from build123d import *

# Parameters (mm, degrees)
SKETCH1_W               = 83.0326
SKETCH1_H               = 17.653
BOSS_EXTRUDE1_DEPTH     = 6.3119
SKETCH5_W               = 2.286
SKETCH5_H               = 21.717
BOSS_EXTRUDE5_DEPTH     = 10.8712
LPATTERN2_COUNT         = 8
LPATTERN2_PITCH         = 9.445171429
SKETCH9_R               = 2.032
CUT_EXTRUDE1_DEPTH      = 86.567236542
MIRROR2_COPY_1_SKETCH_R = 2.032
MIRROR2_COPY_1_DEPTH    = 86.567236542


with BuildPart() as part:
    # Sketch1 → Boss-Extrude1 (new body)
    with BuildSketch(Plane(origin=(0, 0, 0), x_dir=(1, 0, 0), z_dir=(0, 1, 0))):
        with Locations((41.5163, 8.8265)):
            Rectangle(SKETCH1_W, SKETCH1_H)
    extrude(amount=BOSS_EXTRUDE1_DEPTH)

    # Sketch5 → Boss-Extrude5 (add)
    with BuildSketch(Plane.XZ):
        with Locations((8.4582, -8.8265)):
            Rectangle(SKETCH5_W, SKETCH5_H)
    boss_extrude5 = extrude(amount=-BOSS_EXTRUDE5_DEPTH)

    # LPattern2: Boss-Extrude5 ×8
    with Locations(*[(i * LPATTERN2_PITCH, 0, 0) for i in range(1, LPATTERN2_COUNT)]):
        add(boss_extrude5)

    # Sketch9 → Cut-Extrude1 (cut, through all)
    with BuildSketch(Plane(origin=(0, 6.3119, 0), x_dir=(1, 0, 0), z_dir=(0, 1, 0))):
        with Locations(Location((3.3401, 5.08, 0), (0, 0, 270))):
            Circle(SKETCH9_R)
    cut_extrude1 = extrude(amount=-CUT_EXTRUDE1_DEPTH, mode=Mode.SUBTRACT)

    # Mirror1: Cut-Extrude1 across plane
    add(cut_extrude1.mirror(Plane.XY.offset(-8.8265)), mode=Mode.SUBTRACT)

    # Mirror2: Cut-Extrude1 across plane
    add(cut_extrude1.mirror(Plane.ZY.offset(-41.5163)), mode=Mode.SUBTRACT)

    # Mirror2 copy 1 sketch → Mirror2 copy 1 (cut, through all)
    with BuildSketch(Plane(origin=(83.0326, 6.3119, -17.653), x_dir=(-1, 0, 0), z_dir=(0, 1, 0))):
        with Locations(Location((3.3401, 5.08, 0), (0, 0, 270))):
            Circle(MIRROR2_COPY_1_SKETCH_R)
    extrude(amount=-MIRROR2_COPY_1_DEPTH, mode=Mode.SUBTRACT)


solid = part.part
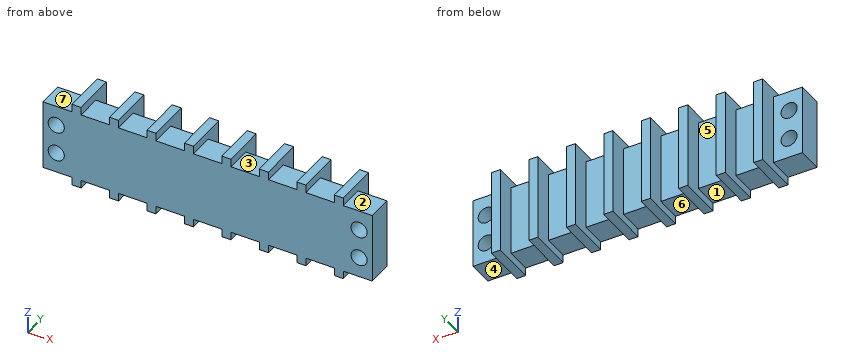
Source: CAD feature listing. Evaluate the final solid. Frame: model axes, mm. Face numbers are marked on the shaded views. A direction names the side the tool comes from. Round coordinates to 2 decimals unless told otherwise and drop trailing zeros. Loops run counter-clockwise (first coordinate to the right, second up) from the corner with the lowest first, then second, coordinate; pieces in that order, holes last. Notation, with made-up numbers: M 12,-20.5 L 56,-20.5 A35 ccw 56,15.5 Z; hole C 85.5,18.25 d3. An arc over 180 degrees is marked long. Answer as CSV lines item,"result".
Q1. Pull-direction query (X, two-part tool) for the marked faces 1 and 2; classes: +X half, -X half, draft (parallel to the pull), parting line (faces both ways), or undercut.
Verdict:
face 1,"undercut"
face 2,"draft"
Q2. Cut plane A-A (z = -5.08). Count the separate pieces of the cut face and the enclosed holes in it, plus the area to 3 significant figures.
Verdict:
separate pieces,"3"
enclosed holes,"0"
area,"556 mm^2"
Q3. Reachability of the marked faces 3, 4, 5, 6 and 7 from +Z, -Z, +X, -X, +Y, -Y: full face, straight path, thin tool, end or side. Return the list, or none.
Verdict:
face 3,"+Z, +Y, -Y"
face 4,"-Z, +X, +Y, -Y"
face 5,"+Z, -Z, +Y"
face 6,"-Z, +Y, -Y"
face 7,"+Z, -X, +Y, -Y"
Q4. Cut plane B-B (x = 30). Return the cut outline in (y, z), plus the area to 3 significant figures.
Verdict:
outline,"M 0,-17.65 L 6.31,-17.65 L 6.31,0 L 0,0 Z"
area,"111 mm^2"
Q5. Contact query for flat-ended pins moving along their axis: pin 1 (5 mm diameter, centred on x = 2, y = 2.5, fed in from +Z); pin 2 (3.5 mm diameter, centred on x = 2, z = -6.5, fed in from +Y); pin 3 (3 mm diameter, centred on x = 70, y = 2.5, fed in from -Z). Output: stop coordinate, or through.
Verdict:
pin 1,"stops at z = 0"
pin 2,"stops at y = 6.31"
pin 3,"stops at z = -17.65"
Q6. Line query: line 1 along X through (y, z) = (3.5, -5.08); line 2 along X through (y, z) = (5.5, -12.25); line 3 along Z through (x, y) = (4, 2.5). Output: solid intervals per line, ascending.
Verdict:
line 1,"x = 0 to 1.31, 5.37 to 77.66, 81.72 to 83.03"
line 2,"x = 0 to 1.33, 5.35 to 77.69, 81.7 to 83.03"
line 3,"z = -17.65 to -14.49, -10.65 to -7, -3.16 to 0"
